Check sheet for the modelled part. Datum: model origin and axes. Units: mm. A direction names the side the tool comes from. Round coordinates to 2 decimals unless told otherwise and drop trailing zeros. Loops run counter-clockwise (first coordinate to the right, second up) from the corner with the lowest first, then second, coordinate; pieces in that order, holes last. Notation, with made-up numbers: M 10,39 L 27,39 A15 ccw 27,61 Z; hole C 35.25,87 d6. An arc over 180 degrees is marked long. One line per question, with ' | ' between items. Start each with the question number.
(1) Section check A-A (z = 53). Record the boundary of the cut face in (x, y).
(2) Thickness scan on probe 1 along Z at (x, y) = (-6, 11); probe 2 along X at (y, z) = (10, 10.5); probe 3 along Y at (x, z) = (23.5, 3.5). Record the ranges inside material, lowest first. Write a range as [from, to].
(3) Go/stop test with a flat-tipped pin: P1, Ø1.5, axis at x = 1, y = 24.5, coming from the -Z side. Record where the tip stops, or that it passes through.
(4) Tool access check on faces 5 (the face through (-1, 0, 29)), 6 (the face through (-21.619, 43, 53)), 7 (the face through (24, 40, 52)). Record the directions out of +Z, -Z, +X, -X, +Y, -Y that give a thin tool (end or side, any length) a straight path to the whole face; none if there is none.
(5) Section check B-B (z = 12). Record the boundary of the cut face in (x, y).
(6) Section check C-C (x = 14). Record the boundary of the cut face in (y, z), and give its area (3 significant figures).
(7) Draft check along X on faces 1 (the face through (26.488, 42.958, 3.521)), 2 (the face through (-21.619, 43, 3)), 3 (the face through (29.381, 23, 28)), 4 (the face through (-29.619, 23, 28)). Enter one of: +X half, -X half, draft (parallel to the pull), parting line (faces both ways), or undercut.
(8) Section check D-D (y = 24). Record the boundary of the cut face in (x, z).
```python
from build123d import *

# Parameters (mm, degrees)
F0_R     = 12
F0_W     = 6
F0_H     = 6
F1_DEPTH = 2
F2_DEPTH = 57
F3_W     = 55
F3_H     = 2
F4_DEPTH = 46
F5_DEPTH = 8
F6_START = 49
F6_DEPTH = 6
F8_START = -28.2
F7_R     = 1.25
F8_DEPTH = 30.8
F9_R     = 3


with BuildPart() as f1:
    # F0 (on Top) → F1 (new body)
    with BuildSketch(Plane.XY):
        Polygon((-27.6188791469, 46), (-29.6188791469, 46), (-29.6188791469, 0), (29.3811208531, 0), (29.3811208531, 46), (27.3811208531, 46), (27.3811208531, 40), (27.3811208531, 2), (-27.6188791469, 2), (-27.6188791469, 40), align=None)
        Polygon((21.3811208531, 46), (-21.6188791469, 46), (-21.6188791469, 40), (-27.6188791469, 40), (-27.6188791469, 2), (27.3811208531, 2), (27.3811208531, 40), (21.3811208531, 40), align=None)
        with Locations((0.0188835789, 24)):
            Circle(F0_R, mode=Mode.SUBTRACT)
        with Locations((-24.6188791469, 43)):
            Rectangle(F0_W, F0_H)
        with Locations((24.3811208531, 43)):
            Rectangle(F0_W, F0_H)
    extrude(amount=F1_DEPTH)

    # F0 (on Top) → F2 (join)
    with BuildSketch(Plane.XY):
        Polygon((-27.6188791469, 46), (-29.6188791469, 46), (-29.6188791469, 0), (29.3811208531, 0), (29.3811208531, 46), (27.3811208531, 46), (27.3811208531, 40), (27.3811208531, 2), (-27.6188791469, 2), (-27.6188791469, 40), align=None)
    extrude(amount=F2_DEPTH)

    # F3 (on Front) → F4 (join)
    with BuildSketch(Plane.XZ):
        with Locations((-0.1188791469, 56)):
            Rectangle(F3_W, F3_H)
    extrude(amount=-F4_DEPTH)

    # F0 (on Top) → F5 (join)
    with BuildSketch(Plane.XY):
        with Locations((24.3811208531, 43)):
            Rectangle(F0_W, F0_H)
        with Locations((-24.6188791469, 43)):
            Rectangle(F0_W, F0_H)
    extrude(amount=F5_DEPTH)

    # F0 (on Top) → F6 (join)
    with BuildSketch(Plane.XY.offset(F6_START)):
        with Locations((24.3811208531, 43)):
            Rectangle(F0_W, F0_H)
        with Locations((-24.6188791469, 43)):
            Rectangle(F0_W, F0_H)
    extrude(amount=F6_DEPTH)

    # F7 (on Front) → F8 (cut)
    with BuildSketch(Plane.XZ.offset(F8_START)):
        with Locations((25.3331962228, 53)):
            Circle(F7_R)
        with Locations((-25.6668037772, 53)):
            Circle(F7_R)
        with Locations((-25.6668037772, 4)):
            Circle(F7_R)
        with Locations((25.3331962228, 4)):
            Circle(F7_R)
    extrude(amount=-F8_DEPTH, mode=Mode.SUBTRACT)

    # F9
    f9_edges = [f1.edges().sort_by_distance(p)[0] for p in [
        (21.381121, 43, 49),
        (-21.618879, 43, 49),
        (-21.618879, 43, 8),
        (21.381121, 43, 8),
    ]]
    fillet(f9_edges, radius=F9_R)


solid = f1.part
```
The answers:
1) outline: M -29.62,0 L 29.38,0 L 29.38,46 L 26.58,46 L 26.58,40 L 27.38,40 L 27.38,2 L -27.62,2 L -27.62,40 L -26.92,40 L -26.92,46 L -29.62,46 Z; M -24.42,40 L -21.62,40 L -21.62,46 L -24.42,46 Z; M 21.38,40 L 24.08,40 L 24.08,46 L 21.38,46 Z
2) probe 1: [0, 2], [55, 57] | probe 2: [-29.62, -27.62], [27.38, 29.38] | probe 3: [0, 2], [40, 46]
3) P1: z = 55
4) face 5: +Z, -Z, +X, -X, -Y | face 6: +Y | face 7: none
5) outline: M -29.62,0 L 29.38,0 L 29.38,46 L 27.38,46 L 27.38,2 L -27.62,2 L -27.62,46 L -29.62,46 Z
6) outline: M 0,0 L 46,0 L 46,2 L 2,2 L 2,55 L 46,55 L 46,57 L 0,57 Z | area: 290 mm²
7) face 1: undercut | face 2: undercut | face 3: +X half | face 4: -X half
8) outline: M -29.62,0 L -11.98,0 L -11.98,2 L -27.62,2 L -27.62,55 L 27.38,55 L 27.38,2 L 12.02,2 L 12.02,0 L 29.38,0 L 29.38,57 L -29.62,57 Z
